```python
from build123d import *

# Parameters (mm, degrees)
EXTRUDE_START   = -25
SKETCH_1_R      = 9
SKETCH_1_R_2    = 7.5
EXTRUDE_1_DEPTH = 2.5
SKETCH_5_R      = 10
SKETCH_5_R_2    = 7.5
EXTRUDE_5_DEPTH = 27.5
EXTRUDE_START_2 = 27.5
SKETCH_1_3_R    = 9
SKETCH_1_3_R_2  = 7.5
EXTRUDE_6_DEPTH = 2.5


with BuildPart() as part:
    # 草圖1 → 填料-伸長1 (new body)
    with BuildSketch(Plane.XY.offset(EXTRUDE_START)):
        with BuildLine():
            Line((132.302720539, 75.19843017), (136.463425545, 5.322192908))
            ThreePointArc((136.463425545, 5.322192908), (146.327410245, -4.082720481), (156.411202737, 5.086124539))
            Line((156.411202737, 5.086124539), (162.224386326, 74.844327616))
            ThreePointArc((162.224386326, 74.844327616), (147.453702316, 91.088959541), (132.302720539, 75.19843017))
        make_face()
        with Locations((147.276199953, 76.090009814)):
            Circle(SKETCH_1_R, mode=Mode.SUBTRACT)
        with Locations((146.445745154, 5.916579337)):
            Circle(SKETCH_1_R_2, mode=Mode.SUBTRACT)
    extrude(amount=-EXTRUDE_1_DEPTH)

    # 草圖5 → 填料-伸長5 (add, symmetric)
    with BuildSketch(Plane.XY):
        with Locations((146.445745154, 5.916579337)):
            Circle(SKETCH_5_R)
        with Locations((146.445745154, 5.916579337)):
            Circle(SKETCH_5_R_2, mode=Mode.SUBTRACT)
    extrude(amount=EXTRUDE_5_DEPTH, both=True)

    # 草圖1<3> → 填料-伸長6 (add)
    with BuildSketch(Plane.XY.offset(EXTRUDE_START_2)):
        with BuildLine():
            Line((132.302720539, 75.19843017), (136.463425545, 5.322192908))
            ThreePointArc((136.463425545, 5.322192908), (146.327410245, -4.082720481), (156.411202737, 5.086124539))
            Line((156.411202737, 5.086124539), (162.224386326, 74.844327616))
            ThreePointArc((162.224386326, 74.844327616), (147.453702316, 91.088959541), (132.302720539, 75.19843017))
        make_face()
        with Locations((147.276199953, 76.090009814)):
            Circle(SKETCH_1_3_R, mode=Mode.SUBTRACT)
        with Locations((146.445745154, 5.916579337)):
            Circle(SKETCH_1_3_R_2, mode=Mode.SUBTRACT)
    extrude(amount=-EXTRUDE_6_DEPTH)


solid = part.part
```
The model under review builds one solid part; all positions refer to its coordinate system, in mm. Round coordinates to 2 decimals unless told otherwise and drop trailing zeros. Loops run counter-clockwise (first coordinate to the right, second up) from the corner with the lowest first, then second, coordinate; pieces in that order, holes last.
Item 1: Take a section at C-C (x = 140.5). Write out the cut boundary in (y, z), then the cut area to 3 significant figures.
Determined:
outline: (-2.12, -27.5) - (1.35, -27.5) - (1.35, 27.5) - (-2.12, 27.5) - close; (10.49, -27.5) - (70.17, -27.5) - (70.17, -25) - (13.96, -25) - (13.96, 25) - (70.17, 25) - (70.17, 27.5) - (10.49, 27.5) - close; (82.01, -27.5) - (89.47, -27.5) - (89.47, -25) - (82.01, -25) - close; (82.01, 25) - (89.47, 25) - (89.47, 27.5) - (82.01, 27.5) - close
area: 700 mm2
Item 2: Take a section at B-B (x = 135). Write out the cut boundary in (y, z).
Determined:
outline: (29.9, -27.5) - (84.71, -27.5) - (84.71, -25) - (29.9, -25) - close; (29.9, 25) - (84.71, 25) - (84.71, 27.5) - (29.9, 27.5) - close
Item 3: Mouldability with a two-part tool opening along X and no side actions: class faces 1 (the face through (134.354, 40.749, 26.268)), 2 (the face through (138.953, 6.246, -0.385)), 3 (the face through (159.277, 39.477, 26.268)) as released by +X, released by -X, zero draft, split by the parting line, or undercut.
Determined:
face 1: released by -X
face 2: undercut
face 3: released by +X
Item 4: Take a section at D-D (x = 147). Write out the cut boundary in (y, z), then the cut area to 3 significant figures.
Determined:
outline: (-4.07, -27.5) - (-1.56, -27.5) - (-1.56, 27.5) - (-4.07, 27.5) - close; (13.4, -27.5) - (67.09, -27.5) - (67.09, -25) - (15.9, -25) - (15.9, 25) - (67.09, 25) - (67.09, 27.5) - (13.4, 27.5) - close; (85.09, -27.5) - (91.09, -27.5) - (91.09, -25) - (85.09, -25) - close; (85.09, 25) - (91.09, 25) - (91.09, 27.5) - (85.09, 27.5) - close
area: 562 mm2
Item 5: Clearance check with flat-ended pins moving along their axes: pin 1 Ø4 at (y, z) = (11, 16) entering from +X; pin 2 Ø14.5 at (x, y) = (147.28, 76.09) entering from +Z; pin 3 Ø4 at (x, z) = (141.5, 16) entering from -Y. State where each tip first meets the part, or that it passes through.
Determined:
pin 1: stops at x = 155.96
pin 2: passes through
pin 3: stops at y = -3.64
Item 6: Take a section at A-A (y = 2). Write out the cut boundary in (x, z).
Determined:
outline: (137.24, -27.5) - (140.05, -27.5) - (140.05, 27.5) - (137.24, 27.5) - close; (152.84, -27.5) - (155.65, -27.5) - (155.65, 27.5) - (152.84, 27.5) - close
Item 7: For line 1 (Z direction, x = 155.5, y = 36.5); line 2 (Y direction, x = 141.5, z = 25.5); line 3 (X direction, y = 7.5, z = 8.5), list the stretches that pass through material, from the lowest coordinate up.
Determined:
line 1: z = -27.5 to -25, 25 to 27.5
line 2: y = -2.77 to 0.28, 11.55 to 69.19, 82.99 to 89.93
line 3: x = 136.57 to 139.11, 153.78 to 156.32
